Part model, mm, in its own coordinate system. Face numbers are marked on the shaded views. A direction names the side the tool comes from. Round coordinates to 2 decimals unless told otherwise and drop trailing zeros. Write each loop counter-clockwise with the first axis right and the second up, starting at its lowest first coordinate (ties: lowest second). Pieces come first, ordered by that corner, then holes.
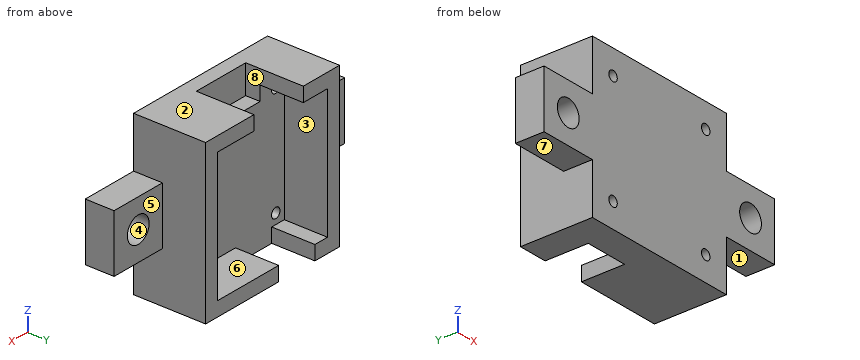
Autodesk Inventor part; units mm, degrees
ref_plane "YZ Plane" through (0, 0, 0) normal (1, 0, 0) x (0, 1, 0)
ref_plane "XZ Plane" through (0, 0, 0) normal (0, 1, 0) x (-1, 0, 0)
ref_plane "XY Plane" through (0, 0, 0) normal (0, 0, 1) x (1, 0, 0)
sketch "스케치1" plane through (0, 0, 0) normal (0, 1, 0) x (-1, 0, 0)
  line L0 (27.717, -55.18) -> (-27.717, -55.18)
  line L1 (-27.717, -55.18) -> (-27.717, 0)
  line L2 (-27.717, 0) -> (27.717, 0)
  line L3 (27.717, 0) -> (27.717, -55.18)
  point P0 (0, 0)
  point P1 (0, 0)
  dimension "d0" = 55.434
  dimension "d1" = 55.18
extrude "돌출1" add sketch "스케치1" along normal blind 5
sketch "스케치2" plane through (0, 5, 0) normal (0, 1, 0) x (1, 0, 0)
  line L0 (-27.717, 0) -> (27.717, 0)
  line L1 (27.717, 0) -> (27.717, 55.18)
  line L2 (27.717, 55.18) -> (-27.717, 55.18)
  line L3 (-27.717, 55.18) -> (-27.717, 0)
  line L4 (-22.717, 50.18) -> (22.717, 50.18)
  line L5 (22.717, 50.18) -> (22.717, 5)
  line L6 (22.717, 5) -> (-22.717, 5)
  line L7 (-22.717, 5) -> (-22.717, 50.18)
  point P0 (0, 0)
  dimension "d4" = 45.434
  dimension "d5" = 45.18
  dimension "d6" = 5
  dimension "d7" = 5
extrude "돌출2" add sketch "스케치2" along normal blind 15
sketch "스케치3" plane through (22.717, 5, -5) normal (0, 0, -1) x (-1, 0, 0)
  line L0 (45.434, 0) -> (0, 0)
  line L1 (45.434, 0) -> (45.434, 15)
  line L2 (0, 15) -> (45.434, 15)
  line L3 (0, 0) -> (0, 15)
  line L4 (15, 15) -> (35.434, 15)
  line L5 (35.434, 15) -> (35.434, 0)
  line L6 (35.434, 0) -> (15, 0)
  line L7 (15, 0) -> (15, 15)
  point P0 (22.717, -5)
  point P1 (15, 0)
  dimension "d10" = 15
  dimension "d11" = 10
extrude "돌출3" cut sketch "스케치3" against normal blind 15 contours L0 L7 L2 L5
sketch "스케치5" plane through (-22.717, 5, -50.18) normal (0, 0, 1) x (1, 0, 0)
  line L0 (45.434, 0) -> (0, 0)
  line L1 (45.434, 0) -> (45.434, 15)
  line L2 (0, 15) -> (45.434, 15)
  line L3 (0, 0) -> (0, 15)
  line L4 (5.2, 15) -> (20.2, 15)
  line L5 (20.2, 15) -> (20.2, 0)
  line L6 (20.2, 0) -> (5.2, 0)
  line L7 (5.2, 0) -> (5.2, 15)
  point P0 (22.717, -5)
  point P1 (5.2, 0)
  dimension "d14" = 15
  dimension "d15" = 5.2
extrude "돌출4" cut sketch "스케치5" against normal blind 10 contours L0 L7 L2 L5
sketch "스케치6" plane through (0, 5, 0) normal (0, 1, 0) x (1, 0, 0)
  line L0 (-22.717, 50.18) -> (-22.717, 5)
  line L1 (-22.717, 5) -> (-12.717, 5)
  line L2 (-12.717, 5) -> (-12.717, 0)
  line L3 (7.717, 0) -> (-12.717, 0)
  line L4 (7.717, 5) -> (7.717, 0)
  line L5 (7.717, 5) -> (22.717, 5)
  line L6 (22.717, 5) -> (22.717, 50.18)
  line L7 (22.717, 50.18) -> (-2.517, 50.18)
  line L8 (-2.517, 50.18) -> (-2.517, 55.18)
  line L9 (-17.517, 55.18) -> (-2.517, 55.18)
  line L10 (-17.517, 50.18) -> (-17.517, 55.18)
  line L11 (-17.517, 50.18) -> (-22.717, 50.18)
  circle A0 centre (-19.177, 46.64) radius 1.75
  circle A1 centre (19.177, 46.64) radius 1.75
  circle A2 centre (-19.177, 8.54) radius 1.75
  circle A3 centre (19.177, 8.54) radius 1.75
  point P0 (0, 0)
  dimension "d18" = 3.5
  dimension "d19" = 3.5
  dimension "d20" = 3.5
  dimension "d21" = 3.5
  dimension "d22" = 3.54
  dimension "d23" = 3.54
  dimension "d24" = 38.354
  dimension "d25" = 38.1
  dimension "d26" = 38.354
  dimension "d27" = 38.1
  dimension "d28" = 3.54
  dimension "d29" = 3.54
  dimension "d30" = 3.54
  dimension "d31" = 3.54
  dimension "d32" = 3.54
  dimension "d33" = 3.54
extrude "돌출5" cut sketch "스케치6" against normal blind 10 contours A0 | A1 | A2 | A3
sketch "스케치7" plane through (27.717, 0, 0) normal (1, 0, 0) x (0, 0, -1)
  line L0 (17.59, 0) -> (37.59, 0)
  line L1 (37.59, 0) -> (37.59, 5)
  line L2 (37.59, 5) -> (17.59, 5)
  line L3 (17.59, 5) -> (17.59, 0)
  line L4 (55.18, 0) -> (55.18, 20)
  line L5 (0, 0) -> (0, 20)
  dimension "d36" = 20
  dimension "d37" = 5
  dimension "d38" = 55.18
  dimension "d39" = 17.59
  dimension "d40" = 15
extrude "돌출6" add sketch "스케치7" along normal blind 20
sketch "스케치8" plane through (27.717, 5, -17.59) normal (0, 1, 0) x (1, 0, 0)
  line L0 (0, 0) -> (0, 20)
  line L1 (0, 0) -> (20, 0)
  line L2 (20, 20) -> (20, 0)
  line L3 (0, 20) -> (20, 20)
  circle A0 centre (10, 10) radius 4.5
  point P0 (-27.717, -17.59)
  dimension "d43" = 9
extrude "돌출7" cut sketch "스케치8" against normal blind 20 contours A0
sketch "스케치9" plane through (-27.717, 0, -55.18) normal (-1, 0, 0) x (0, 0, 1)
  line L0 (17.59, 0) -> (37.59, 0)
  line L1 (37.59, 0) -> (37.59, 5)
  line L2 (37.59, 5) -> (17.59, 5)
  line L3 (17.59, 5) -> (17.59, 0)
  line L4 (55.18, 0) -> (55.18, 20)
  dimension "d46" = 20
  dimension "d47" = 5
  dimension "d48" = 17.59
  dimension "d49" = 15
extrude "돌출8" add sketch "스케치9" along normal blind 20
sketch "스케치10" plane through (-27.717, 5, -17.59) normal (0, 1, 0) x (1, 0, 0)
  line L0 (0, 20) -> (0, 0)
  line L1 (0, 20) -> (-20, 20)
  line L2 (-20, 0) -> (-20, 20)
  line L3 (0, 0) -> (-20, 0)
  circle A0 centre (-10, 10) radius 4.5
  point P0 (27.717, -17.59)
  dimension "d52" = 9
extrude "돌출9" cut sketch "스케치10" against normal blind 20 contours A0
sketch "스케치12" plane through (0, 0, 0) normal (0, -1, 0) x (1, 0, 0)
  circle A0 centre (-37.717, -27.59) radius 4.5
  circle A1 centre (37.717, -27.59) radius 4.5
  circle A2 centre (-19.177, -8.54) radius 1.75
  circle A3 centre (19.177, -46.64) radius 1.75
  circle A4 centre (19.177, -8.54) radius 1.75
  circle A5 centre (-19.177, -46.64) radius 1.75
  line L0 (-27.717, 0) -> (27.717, 0)
  line L1 (-27.717, -17.59) -> (-27.717, 0)
  line L2 (-27.717, -17.59) -> (-47.717, -17.59)
  line L3 (-47.717, -37.59) -> (-47.717, -17.59)
  line L4 (-27.717, -37.59) -> (-47.717, -37.59)
  line L5 (-27.717, -55.18) -> (-27.717, -37.59)
  line L6 (27.717, -55.18) -> (-27.717, -55.18)
  line L7 (27.717, -37.59) -> (27.717, -55.18)
  line L8 (27.717, -37.59) -> (47.717, -37.59)
  line L9 (47.717, -17.59) -> (47.717, -37.59)
  line L10 (27.717, -17.59) -> (47.717, -17.59)
  line L11 (27.717, 0) -> (27.717, -17.59)
  line L12 (-27.717, 0) -> (27.717, 0)
  line L13 (27.717, -55.18) -> (-27.717, -55.18)
  line L14 (27.717, -17.59) -> (47.717, -17.59)
  line L15 (47.717, -17.59) -> (47.717, -37.59)
  line L16 (47.717, -37.59) -> (27.717, -37.59)
  line L17 (-47.717, -17.59) -> (-27.717, -17.59)
  line L18 (-27.717, -37.59) -> (-47.717, -37.59)
  line L19 (-47.717, -37.59) -> (-47.717, -17.59)
  circle A6 centre (-37.717, -27.59) radius 4.5
  circle A7 centre (-19.177, -8.54) radius 1.75
  circle A8 centre (19.177, -8.54) radius 1.75
  circle A9 centre (37.717, -27.59) radius 4.5
  circle A10 centre (19.177, -46.64) radius 1.75
  circle A11 centre (-19.177, -46.64) radius 1.75
  line L20 (-27.717, -55.18) -> (-27.717, -37.59)
  line L21 (-27.717, -17.59) -> (-27.717, 0)
  line L22 (27.717, 0) -> (27.717, -17.59)
  line L23 (27.717, -37.59) -> (27.717, -55.18)
  point P0 (0, 0)
extrude "돌출10" add sketch "스케치12" along normal blind 2
sketch "스케치13" plane through (0, 5, 0) normal (0, 1, 0) x (1, 0, 0)
  circle A0 centre (-19.177, 8.54) radius 1.75
  circle A1 centre (19.177, 46.64) radius 1.75
  circle A2 centre (19.177, 8.54) radius 1.75
  circle A3 centre (-19.177, 46.64) radius 1.75
  line L0 (-22.717, 50.18) -> (-22.717, 5)
  line L1 (-22.717, 5) -> (-12.717, 5)
  line L2 (-12.717, 5) -> (-12.717, 0)
  line L3 (7.717, 0) -> (-12.717, 0)
  line L4 (7.717, 5) -> (7.717, 0)
  line L5 (7.717, 5) -> (22.717, 5)
  line L6 (22.717, 5) -> (22.717, 50.18)
  line L7 (22.717, 50.18) -> (-2.517, 50.18)
  line L8 (-2.517, 50.18) -> (-2.517, 55.18)
  line L9 (-17.517, 55.18) -> (-2.517, 55.18)
  line L10 (-17.517, 50.18) -> (-17.517, 55.18)
  line L11 (-17.517, 50.18) -> (-22.717, 50.18)
  line L12 (-12.717, 0) -> (7.717, 0)
  line L13 (7.717, 0) -> (7.717, 5)
  line L14 (-12.717, 5) -> (-12.717, 0)
  line L15 (7.717, 5) -> (7.717, 10)
  line L16 (7.717, 10) -> (-12.717, 10)
  line L17 (-12.717, 10) -> (-12.717, 5)
  point P0 (0, 0)
  dimension "d57" = 5
extrude "돌출11" cut sketch "스케치13" against normal blind 5 contours L17 L16 L15 L4 L3 L2
sketch "스케치14" plane through (0, -2, 0) normal (0, -1, 0) x (1, 0, 0)
  line L0 (27.717, 0) -> (-27.717, 0)
  line L1 (-27.717, 0) -> (-27.717, -17.59)
  line L2 (-27.717, -17.59) -> (-47.717, -17.59)
  line L3 (-47.717, -17.59) -> (-47.717, -37.59)
  line L4 (-47.717, -37.59) -> (-27.717, -37.59)
  line L5 (-27.717, -37.59) -> (-27.717, -55.18)
  line L6 (-27.717, -55.18) -> (27.717, -55.18)
  line L7 (27.717, -55.18) -> (27.717, -37.59)
  line L8 (27.717, -37.59) -> (47.717, -37.59)
  line L9 (47.717, -37.59) -> (47.717, -17.59)
  line L10 (47.717, -17.59) -> (27.717, -17.59)
  line L11 (27.717, -17.59) -> (27.717, 0)
  circle A0 centre (-37.717, -27.59) radius 4.5
  circle A1 centre (37.717, -27.59) radius 4.5
  circle A2 centre (-19.177, -8.54) radius 1.75
  circle A3 centre (19.177, -46.64) radius 1.75
  circle A4 centre (19.177, -8.54) radius 1.75
  circle A5 centre (-19.177, -46.64) radius 1.75
  line L12 (47.717, -17.59) -> (47.717, -37.59)
  line L13 (-47.717, -37.59) -> (-47.717, -17.59)
  line L14 (-27.717, 0) -> (27.717, 0)
  line L15 (27.717, -55.18) -> (-27.717, -55.18)
  circle A6 centre (-19.177, -8.54) radius 1.75
  circle A7 centre (19.177, -8.54) radius 1.75
  circle A8 centre (19.177, -46.64) radius 1.75
  circle A9 centre (-19.177, -46.64) radius 1.75
  circle A10 centre (-37.717, -27.59) radius 4.5
  circle A11 centre (37.717, -27.59) radius 4.5
  line L16 (-47.717, -17.59) -> (-27.717, -17.59)
  line L17 (27.717, -17.59) -> (47.717, -17.59)
  line L18 (47.717, -37.59) -> (27.717, -37.59)
  line L19 (-27.717, -37.59) -> (-47.717, -37.59)
  line L20 (27.717, 0) -> (27.717, -17.59)
  line L21 (27.717, -37.59) -> (27.717, -55.18)
  line L22 (-27.717, -55.18) -> (-27.717, -37.59)
  line L23 (-27.717, -17.59) -> (-27.717, 0)
  point P0 (0, 0)
extrude "돌출12" add sketch "스케치14" along normal blind 3
properties part number "ZED-F9P-02B-case_new"
Q1. Which spindle directions (+Z, -Z, +X, -X, +Y, -Y) get a long thin tool onto all of the face, cutting with end or side? Do the marked faces 5, 6, 7 and 8. Say none if no direction does.
Values follow:
face 5: +Z, -Z, +X, +Y
face 6: +Y
face 7: -Z, -X, +Y, -Y
face 8: +Z, +Y
Q2. Cut at D-D on y = 1.75. Write the cut outline in (x, z), plus the area to 3 significant figures.
Values follow:
outline: (-47.72, -37.59) - (-27.72, -37.59) - (-27.72, -55.18) - (27.72, -55.18) - (27.72, -37.59) - (47.72, -37.59) - (47.72, -17.59) - (27.72, -17.59) - (27.72, 0) - (7.72, 0) - (7.72, -10) - (-12.72, -10) - (-12.72, 0) - (-27.72, 0) - (-27.72, -17.59) - (-47.72, -17.59) - close; hole circle Ø9 at (-37.72, -27.59); hole circle Ø3.5 at (-19.18, -46.64); hole circle Ø3.5 at (-19.18, -8.54); hole circle Ø3.5 at (19.18, -46.64); hole circle Ø3.5 at (19.18, -8.54); hole circle Ø9 at (37.72, -27.59)
area: 3,490 mm2
Q3. Wall check: L1, parallel to X at y = -1.5, z = -8.54; L2, parallel to X at y = 6.75, z = -30; L3, parallel to X at y = 0.75, z = -27.59. Give the ranges that are in metal, low to high.
Values follow:
L1: x = -27.72 to -20.93, -17.43 to 17.43, 20.93 to 27.72
L2: x = -27.72 to -22.72, 22.72 to 27.72
L3: x = -47.72 to -42.22, -33.22 to 33.22, 42.22 to 47.72
Q4. Drop flat-ended pins along their axis: pin 1 (8 mm diameter, centred on y = 8, z = -2.5, fed in from +X); pin 2 (8 mm diameter, centred on x = 34, y = 0, fed in from -Z); pin 3 (8 mm diameter, centred on y = 9.5, z = -4.5, fed in from -X). Give the stop position or say it passes through.
Values follow:
pin 1: stops at x = 27.72
pin 2: stops at z = -37.59
pin 3: stops at x = -27.72
Q5. Cut at C-C on x = 11.5. Write the cut outline in (y, z).
Values follow:
outline: (-5, -55.18) - (20, -55.18) - (20, -50.18) - (5, -50.18) - (5, -5) - (20, -5) - (20, 0) - (-5, 0) - close
Q6. Mould opens along Z. For the marked faces 1, 2, 3 and 4 say: +Z half, -Z half, draft (parallel to the pull), parting line (faces both ways), or undercut.
Values follow:
face 1: -Z half
face 2: +Z half
face 3: undercut
face 4: undercut
Q7. Cut at B-B on y = 6. Write the cut outline in (x, z).
Values follow:
outline: (-27.72, -55.18) - (-17.52, -55.18) - (-17.52, -50.18) - (-22.72, -50.18) - (-22.72, -5) - (-12.72, -5) - (-12.72, 0) - (-27.72, 0) - close; (-2.52, -55.18) - (27.72, -55.18) - (27.72, 0) - (7.72, 0) - (7.72, -5) - (22.72, -5) - (22.72, -50.18) - (-2.52, -50.18) - close
Q8. Cut at A-A on z = -8.54. Write the cut outline in (x, y).
Values follow:
outline: (-27.72, -5) - (-20.93, -5) - (-20.93, 5) - (-22.72, 5) - (-22.72, 20) - (-27.72, 20) - close; (-17.43, -5) - (17.43, -5) - (17.43, 5) - (7.72, 5) - (7.72, 0) - (-12.72, 0) - (-12.72, 5) - (-17.43, 5) - close; (20.93, -5) - (27.72, -5) - (27.72, 20) - (22.72, 20) - (22.72, 5) - (20.93, 5) - close
